Drawing for the job (mm, zero at the part's lowest x, y, z). A direction names the side the tool comes from. Round coordinates to 2 decimals unless told otherwise and drop trailing zeros. Write each loop counter-clockwise with the first axis right and the second up, starting at its lowest first coordinate (ties: lowest second). Pieces come first, ordered by that corner, then holes.
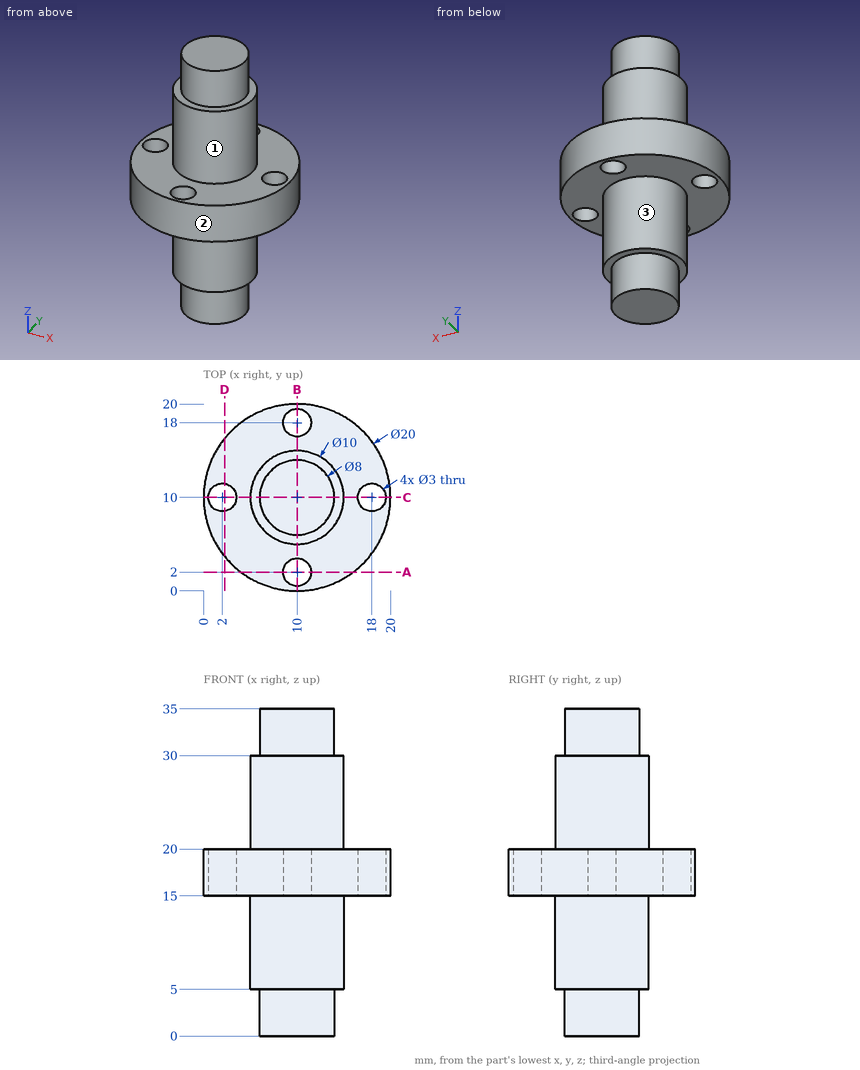
1) Wall check: probe 1 along Z at (x, y) = (6, 5.25); probe 2 along X at (y, z) = (11.25, 19); probe 3 along X at (y, z) = (18, 18.3). Give the ranges that are in metal, low to high.
2) Cut at D-D on x = 2.25. List the corners of the cut face in (y, z), and give its area (3 significant figures).
3) Cut at A-A on y = 2. List the corners of the cut face in (x, z).
4) Flat gauge pins, fed straight in: pin 1 Ø1.5 at (x, z) = (14, 7.5) entering from -Y; pin 2 Ø5 at (x, y) = (18, 10) entering from -Z; pin 3 Ø3 at (x, z) = (7.5, 18.5) entering from -Y. Where does each tip first touch, or does it go through?
5) Which spindle directions (+Z, -Z, +X, -X, +Y, -Y) get a long thin tool onto all of the face, cutting with end or side? Do the marked faces 1, 2 and 3. Say none if no direction does.
6) Cut at B-B on x = 10. List the corners of the cut face in (y, z), and give its area (3 significant figures).
Result sheet:
1. probe 1: z = 15 to 20
1. probe 2: x = 0.08 to 1.17, 2.83 to 17.17, 18.83 to 19.92
1. probe 3: x = 4 to 8.5, 11.5 to 16
2. outline: (3.68, 15) - (8.52, 15) - (8.52, 20) - (3.68, 20) - close; (11.48, 15) - (16.32, 15) - (16.32, 20) - (11.48, 20) - close
2. area: 48.4 mm2
3. outline: (4, 15) - (8.5, 15) - (8.5, 20) - (4, 20) - close; (11.5, 15) - (16, 15) - (16, 20) - (11.5, 20) - close
4. pin 1: stops at y = 6.2
4. pin 2: stops at z = 15
4. pin 3: stops at y = 0.05
5. face 1: +Z
5. face 2: +Z, -Z
5. face 3: -Z
6. outline: (0, 15) - (0.5, 15) - (0.5, 20) - (0, 20) - close; (3.5, 15) - (5, 15) - (5, 5) - (6, 5) - (6, 0) - (14, 0) - (14, 5) - (15, 5) - (15, 15) - (16.5, 15) - (16.5, 20) - (15, 20) - (15, 30) - (14, 30) - (14, 35) - (6, 35) - (6, 30) - (5, 30) - (5, 20) - (3.5, 20) - close; (19.5, 15) - (20, 15) - (20, 20) - (19.5, 20) - close
6. area: 350 mm2
